Here's how the part is built. I have some questions about the finished solid (model axes, mm). Face numbers are marked on the shaded views. A direction names the side the tool comes from. Coordinates: 2 decimals unless noted, no trailing zeros. Order: outer loops, then holes, each group sorted by start corner. A loop starts at its lowest first (then second) coordinate and runs counter-clockwise, first axis right, second up. Notation, with made-up numbers: (-27, 77.5) - (-22, 77.5) arc R19 ccw to (-22, 110.5) - close; hole circle Ø6 at (67.5, -11.5). An arc over 180 degrees is marked (long way). Use CSV: the item, a comma, the result in double quotes. Start each with the question number.
from build123d import *

# Parameters (mm, degrees)
F0_R     = 3
F1_DEPTH = 15
F2_R     = 6
F2_R_2   = 3
F3_DEPTH = 3
F4_SIZE  = 2.99999


# Not quite as in the source:
# - a fillet or chamfer is up to 0.001 mm smaller than in the source, because OpenCascade refuses the exact size


with BuildPart() as f1:
    # F0 (on Right) → F1 (new body)
    with BuildSketch(Plane.YZ):
        Circle(F0_R)
    extrude(amount=F1_DEPTH)

    # F2 (on face) → F3 (join)
    with BuildSketch(Plane.YZ.offset(15)):
        Circle(F2_R)
        Circle(F2_R_2, mode=Mode.SUBTRACT)
    extrude(amount=-F3_DEPTH)

    # F4 (size 3 in the source; OpenCascade refuses exactly that, so slightly less here)
    f4_edges = [f1.edges().sort_by_distance(p)[0] for p in [
        (12, -6, 0),
    ]]
    chamfer(f4_edges, length=F4_SIZE)


solid = f1.part
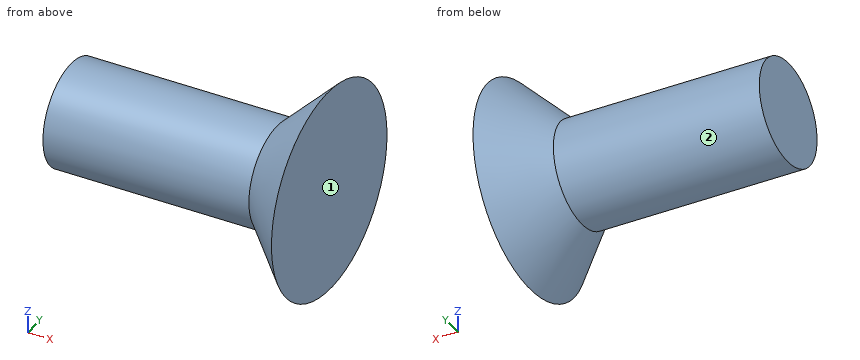
Item 1: Suppose I cut it at C-C on x = 7.75. Write out the boundary of the cut face in (y, z), then the cut area to 3 significant figures.
Item 2: For pin 1 Ø3 at (x, z) = (12.5, -0.5) entering from +Y; pin 2 Ø3 at (x, y) = (8.5, -2) entering from +Z; pin 3 Ø4 at (x, z) = (6, -3) entering from -Y; pin 4 Ø6.5 at (y, z) = (-0.5, -1) entering from -X, each with a flat end and sliding along its axis, tell me the tip position at first contact or that it passes through.
Item 3: Please list where these lines run through material, in increasing order: line 1 along Z through (x, y) = (3.5, 0.25); line 2 along X through (y, z) = (-4, 3.5); line 3 along Z through (x, y) = (11.25, 0.75). Write a range as from..to.
Item 4: For the marked faces 1 and 2, which set-ups out of +Z, -Z, +X, -X, +Y, -Y let a thin tool reach every point of the face, with its end or its side?
Here are the results:
1,outline,"circle Ø6 at (0, 0)"
1,area,"28.3 mm^2"
2,pin 1,"y = 4.98"
2,pin 2,"z = 2.96"
2,pin 3,"y = -2.83"
2,pin 4,"x = 0"
3,line 1,"-2.99..2.99"
3,line 2,"14.32..15"
3,line 3,"-2.9..2.9"
4,face 1,"+Z, -Z, +X, +Y, -Y"
4,face 2,"-X"
